Here's how the part is built. I have some questions about the finished solid (model axes, mm). Coordinates: 2 decimals unless noted, no trailing zeros. Write each loop counter-clockwise with the first axis right and the second up, starting at its lowest first coordinate (ties: lowest second). Pieces come first, ordered by that corner, then holes.
from build123d import *

# Parameters (mm, degrees)
SKETCH1_R                                     = 31.75
BOSS_EXTRUDE1_DEPTH                           = 1.5748
CSK_FOR_4_FLAT_HEAD_SOCKET_CAP_SCREW1_A_COUNT = 2
CSK_FOR_4_FLAT_HEAD_SOCKET_CAP_SCREW1_A_PITCH = 28.575
CSK_FOR_4_FLAT_HEAD_SOCKET_CAP_SCRE_2_COUNT   = 2
CSK_FOR_4_FLAT_HEAD_SOCKET_CAP_SCRE_2_PITCH   = 49.493351826
CSK_FOR_4_FLAT_HEAD_SOCKET_CAP_SCRE_3_COUNT   = 2
CSK_FOR_4_FLAT_HEAD_SOCKET_CAP_SCRE_3_PITCH   = 57.15
CSK_FOR_4_FLAT_HEAD_SOCKET_CAP_SCRE_4_COUNT   = 2
CSK_FOR_4_FLAT_HEAD_SOCKET_CAP_SCRE_4_PITCH   = 49.493351826
CSK_FOR_4_FLAT_HEAD_SOCKET_CAP_SCRE_5_COUNT   = 2
CSK_FOR_4_FLAT_HEAD_SOCKET_CAP_SCRE_5_PITCH   = 28.575


with BuildPart() as part:
    # Sketch1 → Boss-Extrude1 (new body)
    with BuildSketch(Plane(origin=(0, 0, 0), x_dir=(1, 0, 0), z_dir=(0, 1, 0))):
        with Locations(Location((0, 0, 0), (0, 0, 270))):
            Circle(SKETCH1_R)
    extrude(amount=BOSS_EXTRUDE1_DEPTH)

    # Sketch2 → CSK for #4 Flat Head Socket Cap Screw1 (revolve, cut)
    with BuildSketch(Plane(origin=(0, 1.5748, 28.575), x_dir=(0, 0, 1), z_dir=(1, 0, 0))):
        Polygon((0, 0), (0, 1.5748), (1.63195, 1.5748), (1.63195, 1.848124365), (3.2385, 0), align=None)
    csk_for_4_flat_head_socket_cap_screw1 = revolve(axis=Axis((0, 7.9248, 28.575), (0, -1, 0)), mode=Mode.SUBTRACT)

    # CSK for #4 Flat Head Socket Cap Screw1 a: CSK for #4 Flat Head Socket Cap Screw1 ×2
    with Locations(*[Vector(-0.8660254037844382, 0, -0.5000000000000009) * (i * CSK_FOR_4_FLAT_HEAD_SOCKET_CAP_SCREW1_A_PITCH) for i in range(1, CSK_FOR_4_FLAT_HEAD_SOCKET_CAP_SCREW1_A_COUNT)]):
        add(csk_for_4_flat_head_socket_cap_screw1, mode=Mode.SUBTRACT)

    # CSK for _4 Flat Head Socket Cap Scre 2: CSK for #4 Flat Head Socket Cap Screw1 ×2
    with Locations(*[Vector(-0.5000000000000123, 0, -0.8660254037844316) * (i * CSK_FOR_4_FLAT_HEAD_SOCKET_CAP_SCRE_2_PITCH) for i in range(1, CSK_FOR_4_FLAT_HEAD_SOCKET_CAP_SCRE_2_COUNT)]):
        add(csk_for_4_flat_head_socket_cap_screw1, mode=Mode.SUBTRACT)

    # CSK for _4 Flat Head Socket Cap Scre 3: CSK for #4 Flat Head Socket Cap Screw1 ×2
    with Locations(*[(0, 0, -i * CSK_FOR_4_FLAT_HEAD_SOCKET_CAP_SCRE_3_PITCH) for i in range(1, CSK_FOR_4_FLAT_HEAD_SOCKET_CAP_SCRE_3_COUNT)]):
        add(csk_for_4_flat_head_socket_cap_screw1, mode=Mode.SUBTRACT)

    # CSK for _4 Flat Head Socket Cap Scre 4: CSK for #4 Flat Head Socket Cap Screw1 ×2
    with Locations(*[Vector(0.4999999999999877, 0, -0.8660254037844458) * (i * CSK_FOR_4_FLAT_HEAD_SOCKET_CAP_SCRE_4_PITCH) for i in range(1, CSK_FOR_4_FLAT_HEAD_SOCKET_CAP_SCRE_4_COUNT)]):
        add(csk_for_4_flat_head_socket_cap_screw1, mode=Mode.SUBTRACT)

    # CSK for _4 Flat Head Socket Cap Scre 5: CSK for #4 Flat Head Socket Cap Screw1 ×2
    with Locations(*[Vector(0.8660254037844416, 0, -0.499999999999995) * (i * CSK_FOR_4_FLAT_HEAD_SOCKET_CAP_SCRE_5_PITCH) for i in range(1, CSK_FOR_4_FLAT_HEAD_SOCKET_CAP_SCRE_5_COUNT)]):
        add(csk_for_4_flat_head_socket_cap_screw1, mode=Mode.SUBTRACT)


solid = part.part
1. For pin 1 Ø1.5 at (x, z) = (-4.5, 24.5) entering from -Y, with a flat end and sliding along its axis, tell me the tip position at first contact or that it passes through.
2. I want a section at A-A (y = 1.1). State how many separate pieces and enclosed holes the cut face has, then the cut area to 3 significant figures.
3. I want a section at D-D (z = -6). List the corners of the cut face in (x, y) for me.
4. If I drill on line 1 (Z direction, x = -26.5, y = 0.7); line 2 (Z direction, x = 23, y = 0.35); line 3 (Z direction, x = 15, y = 1.25), over which ranges is the centre line in solid material (lowest first)?
Response values:
1. pin 1: stops at y = 0
2. separate pieces: 1
2. enclosed holes: 6
2. area: 3,020 mm2
3. outline: (-31.18, 0) - (31.18, 0) - (31.18, 1.57) - (-31.18, 1.57) - close
4. line 1: z = -17.49 to -16.04, -12.54 to 12.54, 16.04 to 17.49
4. line 2: z = -21.89 to -15.58, -12.99 to 12.99, 15.58 to 21.89
4. line 3: z = -27.98 to 27.98
